Geometry check sheet. Reference: the model listing, model coordinates, mm. Face numbers are marked on the shaded views. A direction names the side the tool comes from. Coordinates: 2 decimals unless noted, no trailing zeros. Loops run counter-clockwise (first coordinate to the right, second up) from the corner with the lowest first, then second, coordinate; pieces in that order, holes last. Notation, with made-up numbers: (-21, 3) -> (14, 3) arc R25 cw to (14, 24) -> close; hole circle Ø6 at (-36, 64). An arc over 180 degrees is marked (long way). Answer as a JSON object with one key per item and string values.
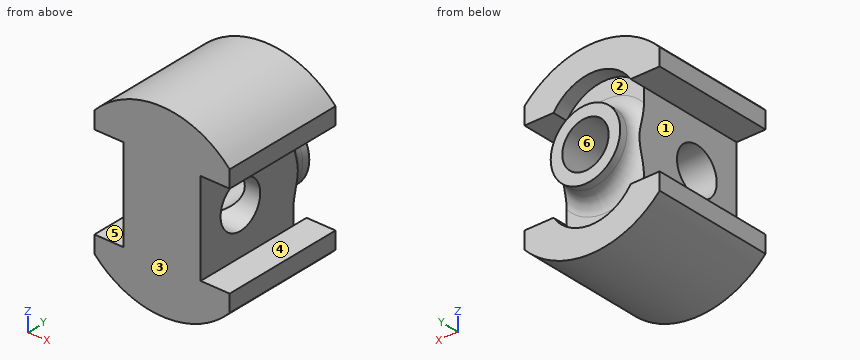
Autodesk Inventor part; units mm, degrees
ref_plane "Work Plane1" through (14.75, 0, 0) normal (1, 0, 0) x (0, 1, 0)
ref_plane "XZ Plane" through (0, 0, 0) normal (0, 1, 0) x (-1, 0, 0)
ref_plane "XY Plane" through (0, 0, 0) normal (0, 0, 1) x (1, 0, 0)
sketch "Sketch1" plane through (0, 0, 0) normal (0, 1, 0) x (-1, 0, 0)
  circle A0 centre (0, 0) radius 12 construction
  line L0 (-5, -16.2951) -> (5, -16.2951) construction
  arc A1 (-8.75, -8.212) -> (8.75, -8.212) centre (0, 0) ccw construction
  arc A2 (-8.75, -8.212) -> (8.75, -8.212) centre (0, 0) ccw
  line L1 (14.6502, 6) -> (14.6502, -6) construction
  line L2 (8.75, -8.212) -> (8.75, -6)
  line L3 (8.75, -6) -> (5, -6)
  line L4 (-8.75, -8.212) -> (-8.75, -6)
  line L5 (-8.75, -6) -> (-5, -6)
  arc A3 (-5, -6) -> (5, -6) centre (0, -2.6834) ccw
  line L6 (14.6502, 0) -> (-10.8345, 0) construction
  line L7 (8.75, -8.212) -> (8.75, 12.1901) construction
  line L8 (-8.75, -8.212) -> (-8.75, 14.7434) construction
  arc A4 (8.75, 8.212) -> (-8.75, 8.212) centre (0, 0) ccw construction
  line L9 (8.75, 8.212) -> (8.75, 6) construction
  arc A5 (8.75, 8.212) -> (-8.75, 8.212) centre (0, 0) ccw
  line L10 (8.75, 8.212) -> (8.75, 6)
  line L11 (-8.75, 8.212) -> (-8.75, 7.106)
  line L12 (-8.75, 7.106) -> (-8.75, 6)
  line L13 (-8.75, 6) -> (-5, 6)
  line L14 (8.75, 6) -> (5, 6)
  arc A6 (5, 6) -> (-5, 6) centre (0, 2.6834) ccw
  line L15 (-5, 6) -> (-5, -6)
  line L16 (5, 6) -> (5, -6)
  circle A7 centre (0, 0) radius 4.75 construction
  circle A8 centre (0, 0) radius 3 construction
  point P0 (0, -16.2951)
  dimension "d0" = 24
  dimension "d1" = 10
  dimension "d2" = 12
  dimension "d3" = 6
  dimension "d4" = 6
  dimension "d5" = 9.5
  dimension "d6" = 6
extrude "Extrusion1" add sketch "Sketch1" along normal blind 16
sketch "Sketch2" plane through (0, 16, 0) normal (0, 1, 0) x (1, 0, 0)
  line L0 (-5, 6) -> (-5, -6)
  line L1 (-5, -6) -> (-5, 6)
  line L2 (5, -6) -> (5, 6)
  line L3 (5, -6) -> (5, 6)
  arc A0 (-5, -6) -> (5, -6) centre (0, -2.6834) ccw
  line L4 (5, 6) -> (8.75, 6)
  arc A1 (5, 6) -> (-5, 6) centre (0, 2.6834) ccw
  point P0 (0, 0)
  dimension "d9" = 6
  dimension "d10" = 6
extrude "Extrusion2" cut sketch "Sketch2" against normal blind 2
sketch "Sketch3" plane through (0, 14, 0) normal (0, 1, 0) x (1, 0, 0)
  circle A0 centre (0, 0) radius 4.5
  circle A1 centre (0, 0) radius 3
  dimension "d13" = 9
  dimension "d14" = 6
extrude "Extrusion3" add sketch "Sketch3" along normal blind 3
fillet "Fillet1" radius 2 1 edges at (-4.5, 14, 0)
ref_plane "Work Plane1" through (14.75, 0, 0) normal (1, 0, 0) x (0, 1, 0)
sketch "Sketch4" plane through (14.75, 0, 0) normal (1, 0, 0) x (0, 1, 0)
  circle A0 centre (6, 0) radius 3
  point P0 (0, 0)
  dimension "d19" = 6
  dimension "d20" = 6
extrude "Extrusion4" cut sketch "Sketch4" against normal blind 888
sketch "Sketch5" plane through (0, 14, 0) normal (0, 1, 0) x (1, 0, 0)
  circle A0 centre (0, 0) radius 3
  dimension "d23" = 6
extrude "Extrusion5" cut sketch "Sketch5" against normal up to surface
thread "Thread2"
properties part number "Crosshead" material "Brass, Soft Yellow"
1. Section check D-D, the plane x = 0. Record the boundary of the cut face in (y, z).
Evaluation:
{"outline": "(0, -12) -> (16, -12) -> (16, -8.68) -> (14, -8.68) -> (14, -6.5) arc R2 cw to (16, -4.5) -> (17, -4.5) -> (17, -3) -> (6, -3) arc R3 cw to (6, 3) -> (17, 3) -> (17, 4.5) -> (16, 4.5) arc R2 cw to (14, 6.5) -> (14, 8.68) -> (16, 8.68) -> (16, 12) -> (0, 12) -> close"}
2. Tool access check on the marked faces 4, 5 and 6. Record the directions out of +Z, -Z, +X, -X, +Y, -Y that give a thin tool (end or side, any length) a straight path to the whole face; none if there is none.
Evaluation:
{"face 4": "+X, +Y, -Y", "face 5": "-X, +Y, -Y", "face 6": "+Y"}
3. Depth check by flat-ended pin: P1, Ø6, axis at y = 4.5, z = 1, coming from the +X side; P2, Ø1, axis at x = -1, y = 4.5, coming from the +Z side; P3, Ø1, axis at x = -4, z = 5, coming from the +Y side. Enter the tip coordinate at first touch or a pass-through.
Evaluation:
{"P1": "stops at x = 5", "P2": "stops at z = 11.99", "P3": "stops at y = 14.09"}
4. Section check B-B, the plane y = 7.5. Record the boundary of the cut face in (x, z).
Evaluation:
{"outline": "(-8.75, -8.21) arc R12 ccw to (8.75, -8.21) -> (8.75, -6) -> (5, -6) -> (5, -2.6) -> (1.5, -2.6) arc R3 cw to (-1.5, -2.6) -> (-5, -2.6) -> (-5, -6) -> (-8.75, -6) -> close; (-8.75, 6) -> (-5, 6) -> (-5, 2.6) -> (-1.5, 2.6) arc R3 cw to (1.5, 2.6) -> (5, 2.6) -> (5, 6) -> (8.75, 6) -> (8.75, 8.21) arc R12 ccw to (-8.75, 8.21) -> close"}
5. Thickness scan on probe 1 along X at (y, z) = (9.5, 0); probe 2 along Z at (x, y) = (0, 13.75); probe 3 along X at (y, z) = (1.5, -5). Record the ranges inside material, lowest first. Write a range as from..to.
Evaluation:
{"probe 1": "x = -5..-3, 3..5", "probe 2": "z = -12..-3, 3..12", "probe 3": "x = -5..5"}
6. Mould release check, pull along X, two halves, no side actions. Record for the marked faces 1, 2 and 3: released by +X, released by -X, zero draft, split by the parting line, or undercut.
Evaluation:
{"face 1": "released by -X", "face 2": "undercut", "face 3": "zero draft"}
7. Section check A-A, the plane z = 0. Record the boundary of the cut face in (x, y).
Evaluation:
{"outline": "(-5, 0) -> (5, 0) -> (5, 3) -> (-5, 3) -> close; (-5, 9) -> (-3, 9) -> (-3, 17) -> (-4.5, 17) -> (-4.5, 16) arc R2 cw to (-5, 14.68) -> close; (3, 9) -> (5, 9) -> (5, 14.68) arc R2 cw to (4.5, 16) -> (4.5, 17) -> (3, 17) -> close"}
8. Section check C-C, the plane x = -7.5. Record the boundary of the cut face in (y, z), then the cut area to 3 significant figures.
Evaluation:
{"outline": "(0, -9.37) -> (16, -9.37) -> (16, -6) -> (0, -6) -> close; (0, 6) -> (16, 6) -> (16, 9.37) -> (0, 9.37) -> close", "area": "108 mm^2"}
